The drawing under review shows one solid part. Ordinate dimensions are in mm from its lowest x, y, z. A direction names the side the tool comes from. Round coordinates to 2 decimals unless told otherwise and drop trailing zeros. Write each loop counter-clockwise with the first axis right and the second up, starting at its lowest first coordinate (ties: lowest second). Pieces come first, ordered by that corner, then holes. Notation, with made-up numbers: (66, 87.5) - (103, 87.5) arc R28 ccw to (103, 115.5) - close; hole circle Ø6 at (20, -16.5). An arc over 180 degrees is marked (long way). Answer in a Markdown table with one row per item. Add a question column.
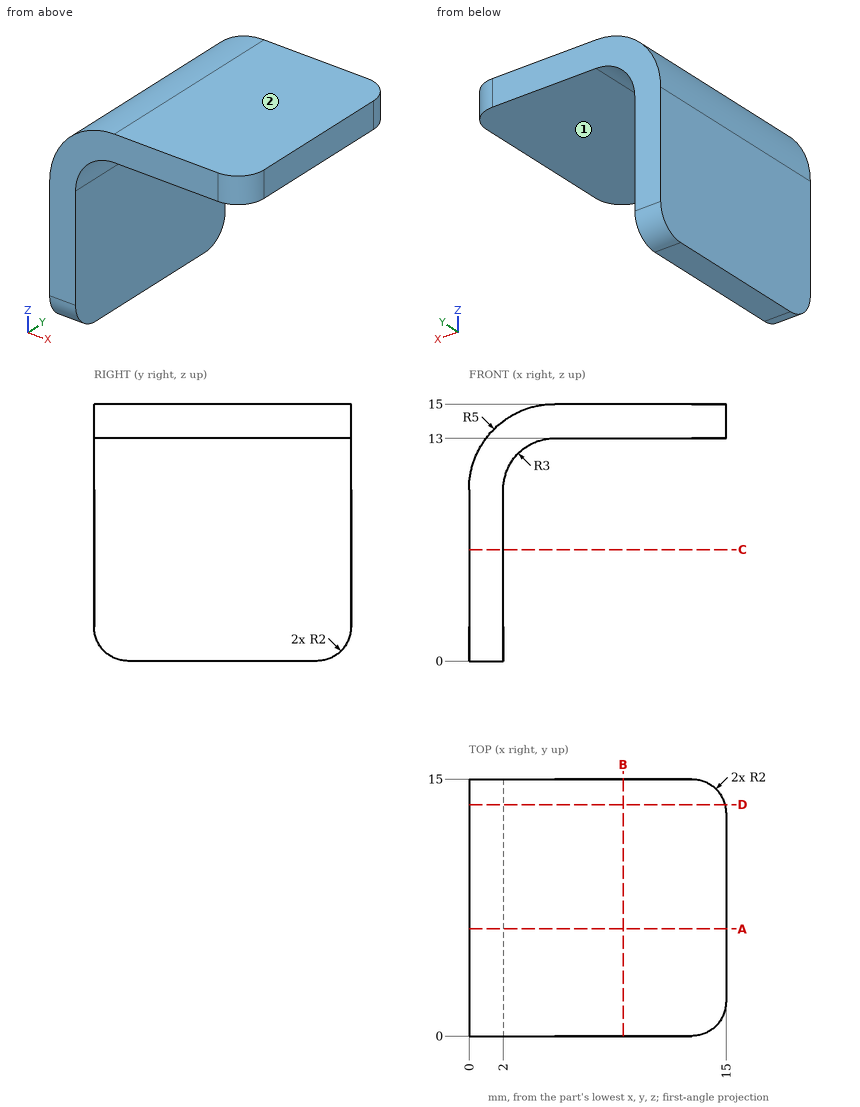
Q1. To check wall thickness, follow probe 1 along X at (y, z) = (4.25, 8); probe 2 along Z at (x, y) = (10.75, 13.5); probe 3 along Z at (x, y) = (2.5, 13.25). State the ranges of each line that lie inside material, in increasing order.
Q2. Add section A-A on y = 6.25. State the section outline as (x, z) points, then the cut area to 3 significant figures.
Q3. Insertion check: pin 1 Ø1.5 at (x, z) = (3, 1.5) entering from -Y; pin 2 Ø1.5 at (x, y) = (4.5, 11) entering from -Z; pin 3 Ø3 at (x, y) = (11.5, 6.5) entering from -Z; pin 4 Ø2 at (x, y) = (4, 4) entering from +Z. Each pin has a flat end and moves straight along its axis. Give the tip position at first contact, or say it passes through.
Q4. Tool access review of the marked faces 1 and 2: name each direction out of +Z, -Z, +X, -X, +Y, -Y from which nothing blocks a thin tool from reaching the whole face with its end or side.
Q5. Add section C-C on z = 6.5. State the section outline as (x, y) points, then the cut area to 3 significant figures.
Q6. Add section B-B on x = 9. State the section outline as (y, z) points, then the cut area to 3 significant figures.
Q7. Add section D-D on y = 13.5. State the section outline as (x, z) points.
Answer sheet:
| question | item | result |
|---|---|---|
| 1 | probe 1 | x = 0 to 2 |
| 1 | probe 2 | z = 13 to 15 |
| 1 | probe 3 | z = 11.66 to 14.33 |
| 2 | outline | (0, 0) - (2, 0) - (2, 10) arc R3 cw to (5, 13) - (15, 13) - (15, 15) - (5, 15) arc R5 ccw to (0, 10) - close |
| 2 | area | 52.6 mm² |
| 3 | pin 1 | passes through |
| 3 | pin 2 | stops at z = 12.73 |
| 3 | pin 3 | stops at z = 13 |
| 3 | pin 4 | stops at z = 15 |
| 4 | face 1 | -Z, +X, +Y, -Y |
| 4 | face 2 | +Z, +X, -X, +Y, -Y |
| 5 | outline | (0, 0) - (2, 0) - (2, 15) - (0, 15) - close |
| 5 | area | 30.0 mm² |
| 6 | outline | (0, 13) - (15, 13) - (15, 15) - (0, 15) - close |
| 6 | area | 30.0 mm² |
| 7 | outline | (0, 0.06) - (2, 0.06) - (2, 10) arc R3 cw to (5, 13) - (14.94, 13) - (14.94, 15) - (5, 15) arc R5 ccw to (0, 10) - close |
